```python
from build123d import *

# Parameters (mm, degrees)
EXTRUDE1_DEPTH     = 609.6
CUT_EXTRUDE1_DEPTH = 51.8


with BuildPart() as part:
    # Sketch1 → Extrude1 (new body)
    with BuildSketch(Plane.XY):
        Polygon((0, 0), (50.8, 0), (50.8, 50.8), (49.2125, 50.8), (49.2125, 1.5875), (0, 1.5875), align=None)
    extrude(amount=EXTRUDE1_DEPTH)

    # Sketch2 → Cut-Extrude1 (cut, through all)
    with BuildSketch(Plane.XZ):
        with BuildLine():
            Line((20.6375, 556.5521), (36.707174868, 556.5521))
            ThreePointArc((36.707174868, 556.5521), (40.809274868, 552.45), (36.707174868, 548.3479))
            Line((36.707174868, 548.3479), (20.6375, 548.3479))
            ThreePointArc((20.6375, 548.3479), (16.5354, 552.45), (20.6375, 556.5521))
        make_face()
        with BuildLine():
            Line((36.707174868, 61.2521), (20.6375, 61.2521))
            ThreePointArc((20.6375, 61.2521), (16.5354, 57.15), (20.6375, 53.0479))
            Line((20.6375, 53.0479), (36.707174868, 53.0479))
            ThreePointArc((36.707174868, 53.0479), (40.809274868, 57.15), (36.707174868, 61.2521))
        make_face()
    extrude(amount=-CUT_EXTRUDE1_DEPTH, mode=Mode.SUBTRACT)


solid = part.part
```
Part model, mm, in its own coordinate system. A direction names the side the tool comes from. Coordinates: 2 decimals unless noted, no trailing zeros. Order: outer loops, then holes, each group sorted by start corner. A loop starts at its lowest first (then second) coordinate and runs counter-clockwise, first axis right, second up. Notation, with made-up numbers: (-8.75, 70) -> (39.25, 70) arc R29 ccw to (39.25, 108) -> close; hole circle Ø11 at (25.25, 66). An arc over 180 degrees is marked (long way). Put each result on its own line as item: value. Start each with the question number.
(1) Probe line 1 along X through (y, z) = (35, 254); line 2 along Y through (x, z) = (10.5, 90). List the from-to ranges inside material, lowest first. Write a range as [from, to].
(2) Band-saw the part on C-C (y = 41.5). Give the cut face in (x, z), then the cut area to 3 significant figures.
(3) Band-saw the part on B-B (x = 7). Give the cut face in (y, z).
(4) Band-saw the part on A-A (z = 375). Give the cut face in (x, y), then the cut area to 3 significant figures.
(5) Which spindle directions (+Z, -Z, +X, -X, +Y, -Y) get a long thin tool onto all of the face, cutting with end or side? Do faces 1 (the face through (50, 14, 609.6)), 2 (the face through (49.212, 27, 301)). Say none if no direction does.
(6) Pin check, flat tips, straight feed: pin 1 Ø3 at (y, z) = (6, 449) entering from -X; pin 2 Ø15 at (x, z) = (34.5, 375.5) entering from +Y. Stop position of each tip, or through.
Determined:
1. line 1: x = [49.21, 50.8]
1. line 2: y = [0, 1.59]
2. outline: (49.21, 0) -> (50.8, 0) -> (50.8, 609.6) -> (49.21, 609.6) -> close
2. area: 968 mm²
3. outline: (0, 0) -> (1.59, 0) -> (1.59, 609.6) -> (0, 609.6) -> close
4. outline: (0, 0) -> (50.8, 0) -> (50.8, 50.8) -> (49.21, 50.8) -> (49.21, 1.59) -> (0, 1.59) -> close
4. area: 159 mm²
5. face 1: +Z, +X, -X, +Y, -Y
5. face 2: +Z, -Z, -X, +Y
6. pin 1: stops at x = 49.21
6. pin 2: stops at y = 1.59
